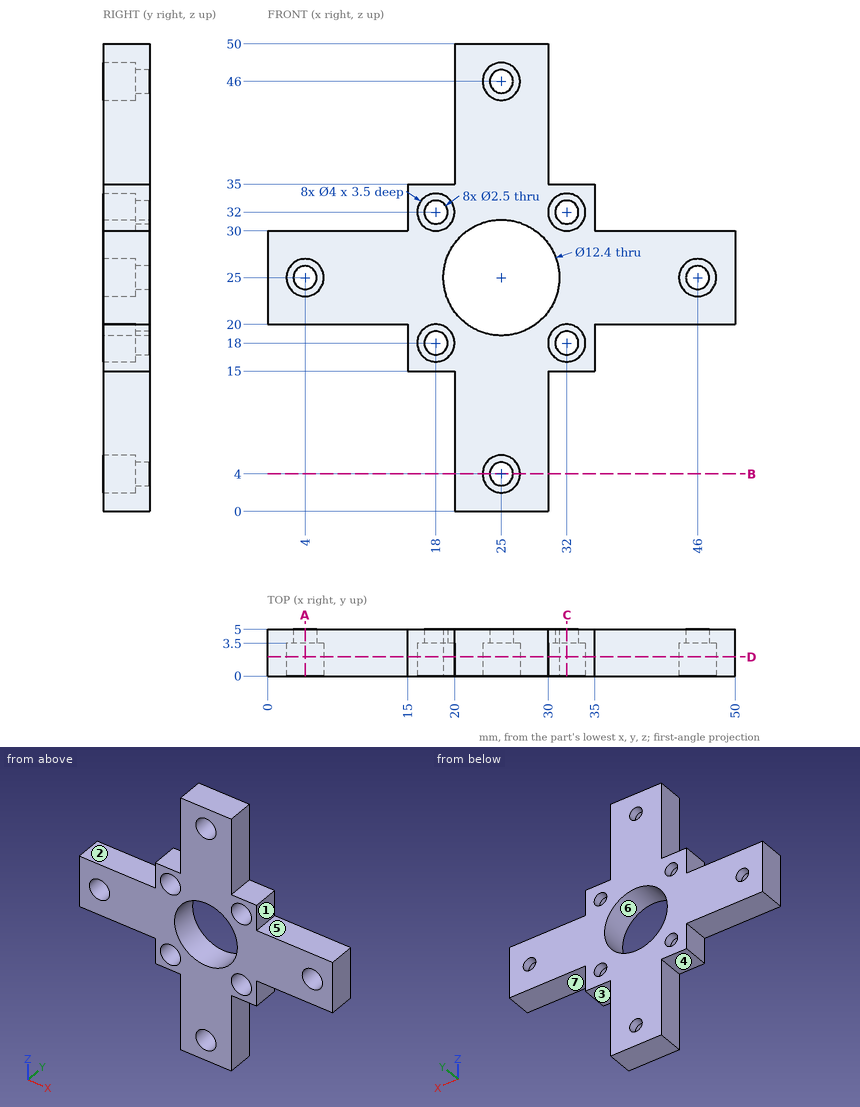
Could you check a few things on this drawing? It's one solid part, dimensions in mm from its lowest x, y, z. A direction names the side the tool comes from. Coordinates: 2 decimals unless noted, no trailing zeros. Loops run counter-clockwise (first coordinate to the right, second up) from the corner with the lowest first, then second, coordinate; pieces in that order, holes last. Notation, with made-up numbers: (-10.75, 27.25) - (17.25, 27.25) arc R6 ccw to (17.25, 35.25) - close; hole circle Ø2 at (-16, 11.5). An arc over 180 degrees is marked (long way). Return JSON: item names as keys, results as strings. Group by question number.
Item 1: I need wall thicknesses on line 1 (X direction, y = 2.15, z = 25); line 2 (X direction, y = 4.1, z = 18); line 3 (Z direction, x = 30.5, y = 0.55). Which ranges of each line are inside material? Lowest first, please. Write a range as from..to.
Item 2: If we section it at A-A on x = 4: Write out the boundary of the cut face in (y, z), and give its area (4 significant figures).
Item 3: If we section it at B-B on z = 4: Write out the boundary of the cut face in (x, y), and give its area (4 significant figures).
Item 4: We'd pull the mould along Z, two halves only. Please class the marked faces 5, 6 and 7: +Z half, -Z half, draft (parallel to the pull), parting line (faces both ways), or undercut.
Item 5: If we section it at D-D on y = 2.05: State how many separate pieces and enclosed holes the cut face has, and give its area (3 significant figures).
Item 6: If we section it at C-C on x = 32: Write out the boundary of the cut face in (y, z).
Item 7: Will these pins go through, and if not, where does the flat tip stop? P1, Ø8, axis at x = 18, z = 39, coming from the +Y side; P2, Ø1.5, axis at x = 31.5, y = 1.5, coming from the +Z side; P3, Ø2.5, axis at y = 2, z = 11, coming from the +X side; P4, Ø1.2, axis at x = 31.5, z = 32.5, coming from the -Y side.
Item 8: On a 3-axis mill with a long thin cutter (end or side, diameter ignored), from which of +Z, -Z, +X, -X, +Y, -Y can I reach the whole of each face in a straight line? I mean the marked faces 1, 2, 3 and 4. Say none if no direction works.
Calculated:
{
 "1": {"line 1": "x = 0..2, 6..18.8, 31.2..44, 48..50", "line 2": "x = 15..16.75, 19.25..30.75, 33.25..35", "line 3": "z = 15..16.68, 19.32..22.14, 27.86..30.68, 33.32..35"},
 "2": {"outline": "(0, 20) - (5, 20) - (5, 23.75) - (3.5, 23.75) - (3.5, 23) - (0, 23) - close; (0, 27) - (3.5, 27) - (3.5, 26.25) - (5, 26.25) - (5, 30) - (0, 30) - close", "area": "32.25 mm^2"},
 "3": {"outline": "(20, 0) - (23, 0) - (23, 3.5) - (23.75, 3.5) - (23.75, 5) - (20, 5) - close; (26.25, 3.5) - (27, 3.5) - (27, 0) - (30, 0) - (30, 5) - (26.25, 5) - close", "area": "32.25 mm^2"},
 "4": {"face 5": "+Z half", "face 6": "undercut", "face 7": "-Z half"},
 "5": {"separate pieces": "1", "enclosed holes": "9", "area": "779 mm^2"},
 "6": {"outline": "(0, 15) - (5, 15) - (5, 16.75) - (3.5, 16.75) - (3.5, 16) - (0, 16) - close; (0, 20) - (3.5, 20) - (3.5, 19.25) - (5, 19.25) - (5, 30.75) - (3.5, 30.75) - (3.5, 30) - (0, 30) - close; (0, 34) - (3.5, 34) - (3.5, 33.25) - (5, 33.25) - (5, 35) - (0, 35) - close"},
 "7": {"P1": "stops at y = 5", "P2": "stops at z = 35", "P3": "stops at x = 30", "P4": "stops at y = 3.5"},
 "8": {"face 1": "+Z, +X, +Y, -Y", "face 2": "+Z, -X, +Y, -Y", "face 3": "-Z, +X, +Y, -Y", "face 4": "-Z, -X, +Y, -Y"}
}
